Model file for the job. Use its own axes, mm. Face numbers are marked on the shaded views. A direction names the side the tool comes from. Give positions to 0.01 mm unless a question says otherwise; leave off trailing zeros. Loops run counter-clockwise (first coordinate to the right, second up) from the corner with the lowest first, then second, coordinate; pieces in that order, holes last. Notation, with made-up numbers: (-10, -4.5) - (44, -4.5) arc R17 cw to (44, 26.5) - close; hole circle Ø5 at (18.5, 16.5). An arc over 180 degrees is marked (long way). Use a Markdown table: item, result.
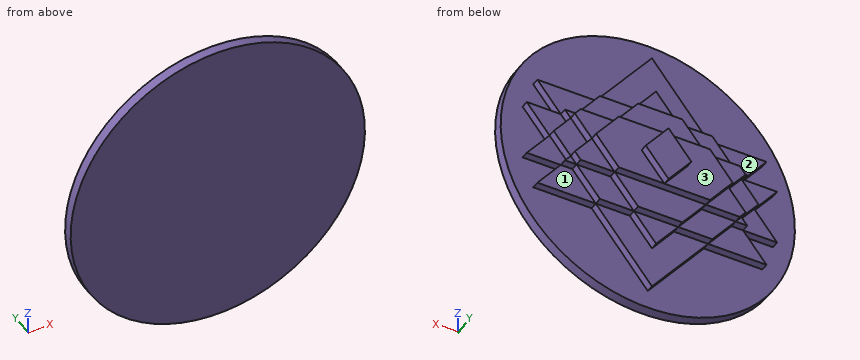
from build123d import *

# Parameters (mm, degrees)
SKETCH1_R            = 300
BOSS_EXTRUDE1_DEPTH  = 10
SKETCH2_R            = 300
BOSS_EXTRUDE2_DEPTH  = 10
BOSS_EXTRUDE4_DEPTH  = 15
BOSS_EXTRUDE5_DEPTH  = 15
BOSS_EXTRUDE11_DEPTH = 15
BOSS_EXTRUDE12_DEPTH = 15
BOSS_EXTRUDE13_DEPTH = 15


with BuildPart() as part:
    # Sketch1 → Boss-Extrude1 (new body)
    with BuildSketch(Plane(origin=(0, 0, 0), x_dir=(1, 0, 0), z_dir=(0, 1, 0))):
        with Locations(Location((0, 0, 0), (0, 0, 270))):
            Circle(SKETCH1_R)
    extrude(amount=-BOSS_EXTRUDE1_DEPTH)

    # Sketch2 → Boss-Extrude2 (add)
    with BuildSketch(Plane.XZ.offset(10)):
        with Locations(Location((0, 0, 0), (0, 0, 90))):
            Circle(SKETCH2_R)
    extrude(amount=BOSS_EXTRUDE2_DEPTH)

    # Sketch3 → Boss-Extrude4 (add)
    with BuildSketch(Plane(origin=(0, 0, 0), x_dir=(1, 0, 0), z_dir=(0, 1, 0))):
        Polygon((-45.133571821, -118.172232568), (-114.539322431, -118.172232568), (0, -261.8), (0, -174.767941529), align=None)
        Polygon((0, -174.767941529), (0, -261.8), (114.539322431, -118.172232568), (45.133571821, -118.172232568), align=None)
        Polygon((233.611993377, -118.172232568), (185.830376799, -58.25598051), (162.32093901, -58.25598051), (114.539322431, -118.172232568), align=None)
        Polygon((255.236127409, -58.25598051), (208.778533209, 0), (174.075657904, -43.516029235), (185.830376799, -58.25598051), align=None)
        Polygon((255.236127409, 58.25598051), (185.830376799, 58.25598051), (174.075657904, 43.516029235), (208.778533209, 0), align=None)
        Polygon((233.611993377, 118.172232568), (114.539322431, 118.172232568), (162.32093901, 58.25598051), (185.830376799, 58.25598051), align=None)
        Polygon((114.539322431, 118.172232568), (0, 261.8), (0, 174.767941529), (45.133571821, 118.172232568), align=None)
        Polygon((0, 174.767941529), (0, 261.8), (-114.539322431, 118.172232568), (-45.133571821, 118.172232568), align=None)
        Polygon((-162.32093901, 58.25598051), (-114.539322431, 118.172232568), (-233.611993377, 118.172232568), (-185.830376799, 58.25598051), align=None)
        Polygon((-174.075657904, 43.516029235), (-185.830376799, 58.25598051), (-255.236127409, 58.25598051), (-208.778533209, 0), align=None)
        Polygon((-174.075657904, -43.516029235), (-208.778533209, 0), (-255.236127409, -58.25598051), (-185.830376799, -58.25598051), align=None)
        Polygon((-162.32093901, -58.25598051), (-185.830376799, -58.25598051), (-233.611993377, -118.172232568), (-114.539322431, -118.172232568), align=None)
        Polygon((-174.075657904, 43.516029235), (-162.32093901, 58.25598051), (-185.830376799, 58.25598051), align=None)
        Polygon((-139.372782599, 0), (-174.075657904, 43.516029235), (-208.778533209, 0), (-174.075657904, -43.516029235), align=None)
        Polygon((-162.32093901, -58.25598051), (-174.075657904, -43.516029235), (-185.830376799, -58.25598051), align=None)
        Polygon((-92.9151884, -58.25598051), (-139.372782599, 0), (-174.075657904, -43.516029235), (-162.32093901, -58.25598051), align=None)
        Polygon((-45.133571821, -118.172232568), (-92.9151884, -58.25598051), (-162.32093901, -58.25598051), (-114.539322431, -118.172232568), align=None)
        Polygon((0, -174.767941529), (0, -118.172232568), (-45.133571821, -118.172232568), align=None)
        Polygon((45.133571821, -118.172232568), (0, -118.172232568), (0, -174.767941529), align=None)
        Polygon((162.32093901, -58.25598051), (92.9151884, -58.25598051), (45.133571821, -118.172232568), (114.539322431, -118.172232568), align=None)
        Polygon((174.075657904, -43.516029235), (139.372782599, 0), (92.9151884, -58.25598051), (162.32093901, -58.25598051), align=None)
        Polygon((185.830376799, -58.25598051), (174.075657904, -43.516029235), (162.32093901, -58.25598051), align=None)
        Polygon((208.778533209, 0), (174.075657904, 43.516029235), (139.372782599, 0), (174.075657904, -43.516029235), align=None)
        Polygon((174.075657904, 43.516029235), (162.32093901, 58.25598051), (92.9151884, 58.25598051), (139.372782599, 0), align=None)
        Polygon((185.830376799, 58.25598051), (162.32093901, 58.25598051), (174.075657904, 43.516029235), align=None)
        Polygon((162.32093901, 58.25598051), (114.539322431, 118.172232568), (45.133571821, 118.172232568), (92.9151884, 58.25598051), align=None)
        Polygon((45.133571821, 118.172232568), (0, 174.767941529), (0, 118.172232568), align=None)
        Polygon((0, 118.172232568), (0, 174.767941529), (-45.133571821, 118.172232568), align=None)
        Polygon((-45.133571821, 118.172232568), (-114.539322431, 118.172232568), (-162.32093901, 58.25598051), (-92.9151884, 58.25598051), align=None)
        Polygon((-92.9151884, 58.25598051), (-162.32093901, 58.25598051), (-174.075657904, 43.516029235), (-139.372782599, 0), align=None)
        Polygon((-46.4575942, 0), (-92.9151884, 58.25598051), (-139.372782599, 0), (-92.9151884, -58.25598051), align=None)
        Polygon((-46.4575942, 0), (0, 58.25598051), (-92.9151884, 58.25598051), align=None)
        Polygon((0, 58.25598051), (0, 118.172232568), (-45.133571821, 118.172232568), (-92.9151884, 58.25598051), align=None)
        Polygon((45.133571821, 118.172232568), (0, 118.172232568), (0, 58.25598051), (92.9151884, 58.25598051), align=None)
        Polygon((92.9151884, 58.25598051), (0, 58.25598051), (46.4575942, 0), align=None)
        Polygon((139.372782599, 0), (92.9151884, 58.25598051), (46.4575942, 0), (92.9151884, -58.25598051), align=None)
        Polygon((92.9151884, -58.25598051), (46.4575942, 0), (0, -58.25598051), align=None)
        Polygon((46.4575942, 0), (0, 0), (0, -58.25598051), align=None)
        Polygon((46.4575942, 0), (0, 58.25598051), (0, 0), align=None)
        Polygon((0, 0), (0, 58.25598051), (-46.4575942, 0), align=None)
        Polygon((0, -58.25598051), (0, 0), (-46.4575942, 0), align=None)
        Polygon((0, -58.25598051), (-46.4575942, 0), (-92.9151884, -58.25598051), align=None)
        Polygon((0, -118.172232568), (0, -58.25598051), (-92.9151884, -58.25598051), (-45.133571821, -118.172232568), align=None)
        Polygon((92.9151884, -58.25598051), (0, -58.25598051), (0, -118.172232568), (45.133571821, -118.172232568), align=None)
    extrude(amount=BOSS_EXTRUDE4_DEPTH)

    # Sketch4 → Boss-Extrude5 (add)
    with BuildSketch(Plane(origin=(0, 15, 0), x_dir=(1, 0, 0), z_dir=(0, 1, 0))):
        Polygon((45.133571821, 118.172232568), (0, 174.767941529), (-45.133571821, 118.172232568), (-114.539322431, 118.172232568), (-162.32093901, 58.25598051), (-185.830376799, 58.25598051), (-174.075657904, 43.516029235), (-208.778533209, 0), (-174.075657904, -43.516029235), (-185.830376799, -58.25598051), (-162.32093901, -58.25598051), (-114.539322431, -118.172232568), (-45.133571821, -118.172232568), (0, -174.767941529), (45.133571821, -118.172232568), (114.539322431, -118.172232568), (162.32093901, -58.25598051), (185.830376799, -58.25598051), (174.075657904, -43.516029235), (208.778533209, 0), (174.075657904, 43.516029235), (185.830376799, 58.25598051), (162.32093901, 58.25598051), (114.539322431, 118.172232568), align=None)
    extrude(amount=BOSS_EXTRUDE5_DEPTH)

    # Sketch6 → Boss-Extrude11 (add)
    with BuildSketch(Plane(origin=(0, 30, 0), x_dir=(1, 0, 0), z_dir=(0, 1, 0))):
        Polygon((0, -118.172232568), (0, -58.25598051), (-92.9151884, -58.25598051), (-45.133571821, -118.172232568), align=None)
        Polygon((92.9151884, -58.25598051), (0, -58.25598051), (0, -118.172232568), (45.133571821, -118.172232568), align=None)
        Polygon((174.075657904, -43.516029235), (139.372782599, 0), (92.9151884, -58.25598051), (162.32093901, -58.25598051), align=None)
        Polygon((139.372782599, 0), (92.9151884, 58.25598051), (46.4575942, 0), (92.9151884, -58.25598051), align=None)
        Polygon((174.075657904, 43.516029235), (162.32093901, 58.25598051), (92.9151884, 58.25598051), (139.372782599, 0), align=None)
        Polygon((45.133571821, 118.172232568), (0, 118.172232568), (0, 58.25598051), (92.9151884, 58.25598051), align=None)
        Polygon((0, 58.25598051), (0, 118.172232568), (-45.133571821, 118.172232568), (-92.9151884, 58.25598051), align=None)
        Polygon((-46.4575942, 0), (-92.9151884, 58.25598051), (-139.372782599, 0), (-92.9151884, -58.25598051), align=None)
        Polygon((-92.9151884, 58.25598051), (-162.32093901, 58.25598051), (-174.075657904, 43.516029235), (-139.372782599, 0), align=None)
        Polygon((-92.9151884, -58.25598051), (-139.372782599, 0), (-174.075657904, -43.516029235), (-162.32093901, -58.25598051), align=None)
        Polygon((0, -58.25598051), (-46.4575942, 0), (-92.9151884, -58.25598051), align=None)
        Polygon((92.9151884, -58.25598051), (46.4575942, 0), (0, -58.25598051), align=None)
        Polygon((46.4575942, 0), (0, 0), (0, -58.25598051), align=None)
        Polygon((0, -58.25598051), (0, 0), (-46.4575942, 0), align=None)
        Polygon((0, 0), (0, 58.25598051), (-46.4575942, 0), align=None)
        Polygon((46.4575942, 0), (0, 58.25598051), (0, 0), align=None)
        Polygon((92.9151884, 58.25598051), (0, 58.25598051), (46.4575942, 0), align=None)
        Polygon((-46.4575942, 0), (0, 58.25598051), (-92.9151884, 58.25598051), align=None)
    extrude(amount=BOSS_EXTRUDE11_DEPTH)

    # Sketch10 → Boss-Extrude12 (add)
    with BuildSketch(Plane(origin=(0, 45, 0), x_dir=(1, 0, 0), z_dir=(0, 1, 0))):
        Polygon((-46.4575942, 0), (-92.9151884, 58.25598051), (-139.372782599, 0), (-92.9151884, -58.25598051), align=None)
        Polygon((-46.4575942, 0), (0, 58.25598051), (-92.9151884, 58.25598051), align=None)
        Polygon((92.9151884, 58.25598051), (0, 58.25598051), (46.4575942, 0), align=None)
        Polygon((139.372782599, 0), (92.9151884, 58.25598051), (46.4575942, 0), (92.9151884, -58.25598051), align=None)
        Polygon((92.9151884, -58.25598051), (46.4575942, 0), (0, -58.25598051), align=None)
        Polygon((46.4575942, 0), (0, 58.25598051), (0, 0), align=None)
        Polygon((0, 0), (0, 58.25598051), (-46.4575942, 0), align=None)
        Polygon((0, -58.25598051), (0, 0), (-46.4575942, 0), align=None)
        Polygon((46.4575942, 0), (0, 0), (0, -58.25598051), align=None)
        Polygon((0, -58.25598051), (-46.4575942, 0), (-92.9151884, -58.25598051), align=None)
    extrude(amount=BOSS_EXTRUDE12_DEPTH)

    # Sketch11 → Boss-Extrude13 (add)
    with BuildSketch(Plane(origin=(0, 60, 0), x_dir=(1, 0, 0), z_dir=(0, 1, 0))):
        Polygon((0, 0), (0, 58.25598051), (-46.4575942, 0), align=None)
        Polygon((46.4575942, 0), (0, 58.25598051), (0, 0), align=None)
        Polygon((46.4575942, 0), (0, 0), (0, -58.25598051), align=None)
        Polygon((0, -58.25598051), (0, 0), (-46.4575942, 0), align=None)
    extrude(amount=BOSS_EXTRUDE13_DEPTH)


solid = part.part
(1) 3-axis set-ups, long thin cutter, end or side, ignore diameter. For the marked faces 1, 2 and 3: which of +Z, -Z, +X, -X, +Y, -Y reach the whole face in a straight line?
Computed:
| item | result |
|---|---|
| face 1 | -Z, +X, +Y |
| face 2 | +Z, -X, +Y |
| face 3 | -X, +Y |
(2) Drill centre lines: probe 1 along Z at (x, y) = (180, 20); probe 2 along Y at (x, z) = (65, 155); probe 3 along Y at (x, z) = (72.5, -89.5). Where is each one in solid material? Low to high. Write a range as [from, to].
Computed:
| item | result |
|---|---|
| probe 1 | [-58.26, -50.94], [-36.09, 36.09], [50.94, 58.26] |
| probe 2 | [-20, 15] |
| probe 3 | [-20, 30] |
(3) Pin check, flat tips, straight feed: P1, Ø16.5, axis at x = -82.5, y = 19, coming from the +Z side; P2, Ø18, axis at x = 81.5, z = 78.5, coming from the +Y side; P3, Ø12, axis at x = 77.5, y = 22, coming from the +Z side. Stop position of each tip, or through.
Computed:
| item | result |
|---|---|
| P1 | z = 167.4 |
| P2 | y = 45 |
| P3 | z = 118.17 |
(4) Slice it at C-C, the plane z = -110. Write the cut outline in (x, y), plus the area to 3 significant figures.
Computed:
| item | result |
|---|---|
| outline | (-279.11, -20) - (279.11, -20) - (279.11, 0) - (227.09, 0) - (227.09, 15) - (121.06, 15) - (121.06, 30) - (51.65, 30) - (51.65, 45) - (-51.65, 45) - (-51.65, 30) - (-121.06, 30) - (-121.06, 15) - (-227.09, 15) - (-227.09, 0) - (-279.11, 0) - close |
| area | 23,200 mm² |
(5) Slice it at D-D, the plane z = 217. Write the cut outline in (x, y).
Computed:
| item | result |
|---|---|
| outline | (-207.15, -20) - (207.15, -20) - (207.15, 0) - (35.73, 0) - (35.73, 15) - (-35.73, 15) - (-35.73, 0) - (-207.15, 0) - close |
(6) Slice it at B-B, the plane x = 9. Write the cut outline in (y, z), plus the area to 3 significant figures.
Computed:
| item | result |
|---|---|
| outline | (-20, -299.86) - (0, -299.86) - (0, -250.51) - (15, -250.51) - (15, -163.48) - (30, -163.48) - (30, -118.17) - (45, -118.17) - (45, -58.26) - (60, -58.26) - (60, -46.97) - (75, -46.97) - (75, 46.97) - (60, 46.97) - (60, 58.26) - (45, 58.26) - (45, 118.17) - (30, 118.17) - (30, 163.48) - (15, 163.48) - (15, 250.51) - (0, 250.51) - (0, 299.86) - (-20, 299.86) - close |
| area | 31,100 mm² |
(7) Slice it at A-A, the plane z = -15. Write the cut outline in (x, y), plus the area to 3 significant figures.
Computed:
| item | result |
|---|---|
| outline | (-299.62, -20) - (299.62, -20) - (299.62, 0) - (220.74, 0) - (220.74, 15) - (196.82, 15) - (196.82, 30) - (151.33, 30) - (151.33, 45) - (127.41, 45) - (127.41, 60) - (34.5, 60) - (34.5, 75) - (-34.5, 75) - (-34.5, 60) - (-127.41, 60) - (-127.41, 45) - (-151.33, 45) - (-151.33, 30) - (-196.82, 30) - (-196.82, 15) - (-220.74, 15) - (-220.74, 0) - (-299.62, 0) - close |
| area | 33,900 mm² |
